Study the drawing (mm; zero at the part's minimum x, y, z) and answer. Give positions to 0.01 mm unless a question says otherwise; leave off trailing zeros. Write each loop counter-clockwise with the first axis right and the second up, starting at its lowest first coordinate (ties: lowest second). Pieces come first, ordered by that corner, then holes. Notation, with made-up numbers: (55, -34.75) -> (88, -34.75) arc R30 ccw to (88, -3.75) -> close; hole circle Ø5 at (45.25, 77). An arc over 180 degrees is marked (long way). One line per question, with ' | ' between items.
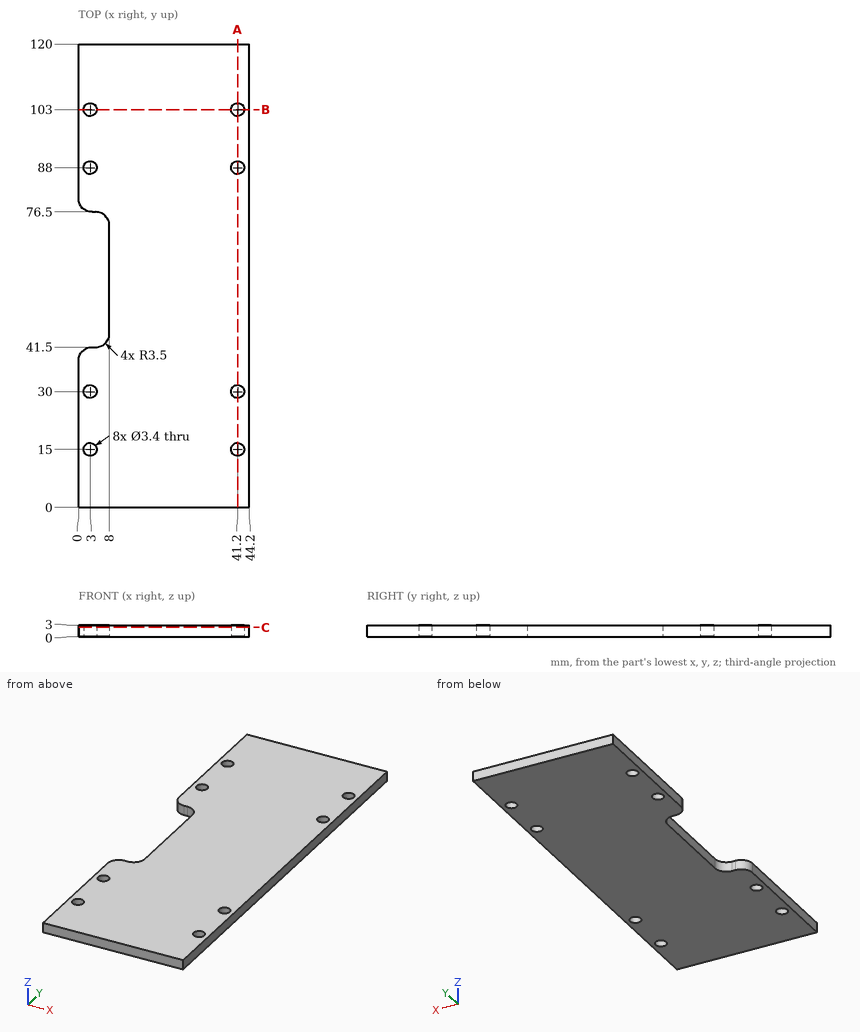
Item 1: Find section B-B (y = 103). Write down the section's boundary in (x, z), then the cut area to 3 significant figures.
Answers below:
outline: (0, 0) -> (1.3, 0) -> (1.3, 3) -> (0, 3) -> close; (4.7, 0) -> (39.5, 0) -> (39.5, 3) -> (4.7, 3) -> close; (42.9, 0) -> (44.2, 0) -> (44.2, 3) -> (42.9, 3) -> close | area: 112 mm²
Item 2: Find section C-C (z = 2.45). Count the separate pieces of the cut face and the enclosed holes in it, then the cut area to 3 significant figures.
Answers below:
separate pieces: 1 | enclosed holes: 8 | area: 4,950 mm²
Item 3: Consider line 1 (Y direction, x = 41.2, z = 2.2); line 2 (X direction, y = 103, z = 0.8); line 3 (X direction, y = 89, z = 2.55). Determine where each line is inside the solid, lowest interval first. Write a range as [from, to].
Answers below:
line 1: [0, 13.3], [16.7, 28.3], [31.7, 86.3], [89.7, 101.3], [104.7, 120] | line 2: [0, 1.3], [4.7, 39.5], [42.9, 44.2] | line 3: [0, 1.63], [4.37, 39.83], [42.57, 44.2]
Item 4: Find section A-A (x = 41.2). Write down the section's boundary in (y, z).
Answers below:
outline: (0, 0) -> (13.3, 0) -> (13.3, 3) -> (0, 3) -> close; (16.7, 0) -> (28.3, 0) -> (28.3, 3) -> (16.7, 3) -> close; (31.7, 0) -> (86.3, 0) -> (86.3, 3) -> (31.7, 3) -> close; (89.7, 0) -> (101.3, 0) -> (101.3, 3) -> (89.7, 3) -> close; (104.7, 0) -> (120, 0) -> (120, 3) -> (104.7, 3) -> close
